Here's the drawing with two shaded views (mm, measured from the low corner). I have some questions. A direction names the side the tool comes from. Coordinates: 2 decimals unless noted, no trailing zeros. Write each loop counter-clockwise with the first axis right and the second up, starting at its lowest first coordinate (ties: lowest second). Pieces come first, ordered by that corner, then holes.
Item 1: Thinking about a two-plate mould opening in Z: for the marked faces 3, 4 and 5, which applies, +Z half, -Z half, draft (parallel to the pull), parting line (faces both ways), or undercut?
Item 2: If I drill on probe 1 along X at (y, z) = (1.85, 15); probe 2 along Y at (x, z) = (10, 2.5); probe 3 along Y at (x, z) = (14.75, 12.25), over which ranges is the centre line in solid material (lowest first)?
Item 3: I want a section at A-A on x = 10.5. Please give me the cut outline in (y, z), then the cut area to 3 significant figures.
Item 4: For P1, Ø6, axis at x = 7, z = 12.5, coming from the +Y side; P2, Ø2, axis at x = 13.5, y = 2, coming from the +Z side; P3, Ø8, axis at x = 13.5, y = 11.5, coming from the +Z side; P4, Ø1.5, axis at x = 11.5, y = 6.5, coming from the -Z side, each with a flat end and sliding along its axis, tell me the tip position at first contact or that it passes through.
Item 5: I want a section at D-D on y = 3.25. Please give me the cut outline in (x, z), then the cut area to 3 significant figures.
Item 6: Which directions (+Z, -Z, +X, -X, +Y, -Y) give clear straight access to the entire face, cutting with the end or side of a thin tool? Please do the marked faces 1 and 2.
Item 7: I want a section at B-B on z = 1.5. Please give me the cut outline in (x, y).
Item 8: I want a section at C-C on y = 10. Please give me the cut outline in (x, z), then the cut area to 3 significant figures.
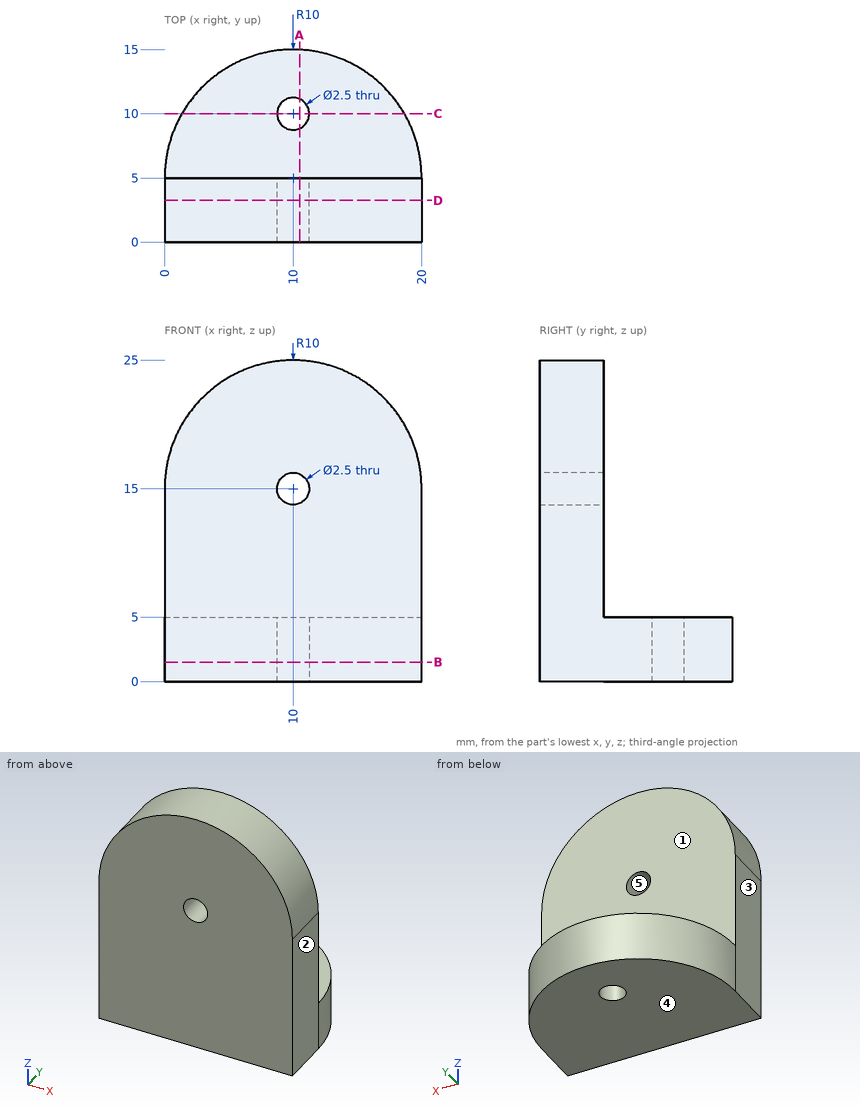
Response values:
1. face 3: draft
1. face 4: -Z half
1. face 5: undercut
2. probe 1: x = 0 to 8.75, 11.25 to 20
2. probe 2: y = 0 to 8.75, 11.25 to 15
2. probe 3: y = 0 to 5
3. outline: (0, 0) - (8.85, 0) - (8.85, 5) - (5, 5) - (5, 13.85) - (0, 13.85) - close; (0, 16.15) - (5, 16.15) - (5, 24.99) - (0, 24.99) - close; (11.15, 0) - (14.99, 0) - (14.99, 5) - (11.15, 5) - close
3. area: 152 mm2
4. P1: stops at y = 5
4. P2: stops at z = 24.68
4. P3: stops at z = 5
4. P4: stops at z = 0
5. outline: (0, 0) - (20, 0) - (20, 15) arc R10 ccw to (0, 15) - close; hole circle Ø2.5 at (10, 15)
5. area: 452 mm2
6. face 1: +Z, +X, -X, +Y
6. face 2: +Z, -Z, +X, +Y, -Y
7. outline: (0, 0) - (20, 0) - (20, 5) arc R10 ccw to (0, 5) - close; hole circle Ø2.5 at (10, 10)
8. outline: (1.34, 0) - (8.75, 0) - (8.75, 5) - (1.34, 5) - close; (11.25, 0) - (18.66, 0) - (18.66, 5) - (11.25, 5) - close
8. area: 74.1 mm2
